Check sheet for the modelled part. Datum: model origin and axes. Units: mm. Round coordinates to 2 decimals unless told otherwise and drop trailing zeros. Order: outer loops, then holes, each group sorted by start corner. A loop starts at its lowest first (then second) coordinate and runs counter-clockwise, first axis right, second up. Notation, with made-up numbers: (67, -7) -> (72, -7) arc R24 ccw to (72, 14) -> close; hole circle Ø8 at (-18, 1). An arc over 180 degrees is marked (long way). Answer in a Markdown table with one row per item.
from build123d import *

# Parameters (mm, degrees)
BASPROSKE_W           = 5
BASPROSKE_H           = 7
TOOTHCUT_DEPTH        = 50.749371855
TEETHCUTS_COUNT       = 30
TEETHCUTS_ANGLE       = 348
CROQUIS1_OUTSIDE_W    = 91.824
CROQUIS1_OUTSIDE_H    = 91.824
CROQUIS1_OUTSIDE_R    = 33
CORTAR_EXTRUIR1_DEPTH = 50.749371855


with BuildPart() as part:
    # BasProSke → Base-Revolve (revolve)
    with BuildSketch(Plane(origin=(0, 0, 0), x_dir=(1, 0, 0), z_dir=(0, 1, 0)), mode=Mode.PRIVATE) as base_revolve_sk:
        with Locations((2.5, 31.5)):
            Rectangle(BASPROSKE_W, BASPROSKE_H)
    revolve(base_revolve_sk.sketch.rotate(Axis((-10, 0, 0), (1, 0, 0)), 180), axis=Axis((-10, 0, 0), (1, 0, 0)))

    # TooCutSke → ToothCut (cut, through all)
    with BuildSketch(Plane(origin=(0, 0, 0), x_dir=(0, 0, -1), z_dir=(1, 0, 0))):
        with BuildLine():
            ThreePointArc((2.421581378, 27.869592548), (1.601037152, 30.270461464), (0.387584664, 32.498688883))
            ThreePointArc((0.387584664, 32.498688883), (0, 32.501), (-0.387584664, 32.498688883))
            ThreePointArc((-0.387584664, 32.498688883), (-1.601037152, 30.270461464), (-2.421581378, 27.869592548))
            ThreePointArc((-2.421581378, 27.869592548), (0, 27.9746), (2.421581378, 27.869592548))
        make_face()
    toothcut = extrude(amount=TOOTHCUT_DEPTH, mode=Mode.SUBTRACT)

    # TeethCuts: ToothCut ×30 about axis
    teethcuts_axis = Axis((-10, 0, 0), (1, 0, 0))
    for i in range(1, TEETHCUTS_COUNT):
        add(toothcut.rotate(teethcuts_axis, i * TEETHCUTS_ANGLE / (TEETHCUTS_COUNT - 1)), mode=Mode.SUBTRACT)

    # Croquis1 outside → Cortar-Extruir1 (cut, through all)
    with BuildSketch(Plane(origin=(5, 0, 0), x_dir=(0, 0, -1), z_dir=(1, 0, 0))):
        Rectangle(CROQUIS1_OUTSIDE_W, CROQUIS1_OUTSIDE_H)
        Circle(CROQUIS1_OUTSIDE_R, mode=Mode.SUBTRACT)
    extrude(amount=-CORTAR_EXTRUIR1_DEPTH, mode=Mode.SUBTRACT)


solid = part.part
Item 1: Cross-section at B-B (y = -23). Record the boundary of the cut face in (x, z).
Result sheet:
| item | result |
|---|---|
| outline | (0, -23.66) -> (5, -23.66) -> (5, -18.96) -> (0, -18.96) -> close; (0, 18.96) -> (5, 18.96) -> (5, 23.66) -> (0, 23.66) -> close |
Item 2: Mould release check, pull along Z, two halves, no side actions. Record for faces 1 (the flat face through (5, 24.3, -14.5)), 2 (the cylindrical face through (2.46, -10.88, -28.27)), 3 (the cylindrical face through (2.46, 13.73, -27)), 4 (the cylindrical face through (2.5, -12.6, -30.5)): pulls with the +Z half, pulls with the -Z half, needs draft (parallel to the pull), parting line crosses it, or undercut.
Result sheet:
| item | result |
|---|---|
| face 1 | needs draft |
| face 2 | undercut |
| face 3 | undercut |
| face 4 | parting line crosses it |
Item 3: Cross-section at A-A (z = -5). Record the boundary of the cut face in (x, y), and give its area (3 significant figures).
Result sheet:
| item | result |
|---|---|
| outline | (0, -32.62) -> (5, -32.62) -> (5, -30.31) -> (0, -30.31) -> close; (0, 30.31) -> (5, 30.31) -> (5, 32.62) -> (0, 32.62) -> close |
| area | 23.1 mm^2 |
Item 4: Depth check by flat-ended pin: P1, Ø5, axis at y = 24, z = 2.5, coming from the -X side; P2, Ø3, axis at x = 2.5, z = 11.5, coming from the +Y side. Enter the tip coordinate at first touch or a pass-through.
Result sheet:
| item | result |
|---|---|
| P1 | passes through |
| P2 | stops at y = 31.45 |
Item 5: Scan lines: line 1 (Z direction, x = 1.55, y = 28.5); line 2 (Y direction, x = 1.5, z = 23); line 3 (Z direction, x = 4.8, y = -29.5). Record each from-to range of solid material in increasing order. Write a range as [from, to].
Result sheet:
| item | result |
|---|---|
| line 1 | z = [-16.64, -13.71], [-11.07, -8], [-3.81, -2.25], [2.25, 3.81], [8, 11.07], [13.71, 16.64] |
| line 2 | y = [-23.66, -21.87], [-17.94, -16.05], [16.05, 17.94], [21.87, 23.66] |
| line 3 | z = [-14.79, -13.58], [-12.35, -7.81], [-4.42, -1.91], [1.91, 4.42], [7.81, 12.35], [13.58, 14.79] |
